CAD build for the part. Positions are in the model's coordinates, mm. Coordinates: 2 decimals unless noted, no trailing zeros. Order: outer loops, then holes, each group sorted by start corner. A loop starts at its lowest first (then second) coordinate and runs counter-clockwise, first axis right, second up. Notation, with made-up numbers: (11, 74.5) - (54, 74.5) arc R32 cw to (54, 113.5) - close; hole circle Ø10 at (59.5, 51). An arc over 180 degrees is marked (long way). Use one line per item in the form item = value.
```python
from build123d import *

# Parameters (mm, degrees)
F0_R     = 10
F1_DEPTH = 50
F2_DEPTH = 75
F3_SIZE  = 2


with BuildPart() as f1:
    # F0 (on Front) → F1 (new body)
    with BuildSketch(Plane.XZ):
        with BuildLine():
            ThreePointArc((2.083333, 24.913043), (18.399502, 16.92508), (25, 0))
            ThreePointArc((25, 0), (18.399502, -16.92508), (2.083333, -24.913043))
            Line((2.083333, -24.913043), (91.458333, -17.43913))
            ThreePointArc((91.458333, -17.43913), (72.5, 0), (91.458333, 17.43913))
            Line((91.458333, 17.43913), (2.083333, 24.913043))
        make_face()
        with BuildLine():
            ThreePointArc((2.083333, -24.913043), (18.399502, -16.92508), (25, 0))
            ThreePointArc((25, 0), (18.399502, 16.92508), (2.083333, 24.913043))
            ThreePointArc((2.083333, 24.913043), (-25, 0), (2.083333, -24.913043))
        make_face()
        Circle(F0_R, mode=Mode.SUBTRACT)
        with BuildLine():
            ThreePointArc((107.5, 0), (102.879651, 11.847556), (91.458333, 17.43913))
            ThreePointArc((91.458333, 17.43913), (72.5, 0), (91.458333, -17.43913))
            ThreePointArc((91.458333, -17.43913), (102.879651, -11.847556), (107.5, 0))
        make_face()
        with Locations((90, 0)):
            Circle(F0_R, mode=Mode.SUBTRACT)
    extrude(amount=F1_DEPTH)

    # F0 (on Front) → F2 (join)
    with BuildSketch(Plane.XZ):
        with BuildLine():
            ThreePointArc((2.083333, -24.913043), (18.399502, -16.92508), (25, 0))
            ThreePointArc((25, 0), (18.399502, 16.92508), (2.083333, 24.913043))
            ThreePointArc((2.083333, 24.913043), (-25, 0), (2.083333, -24.913043))
        make_face()
        Circle(F0_R, mode=Mode.SUBTRACT)
        with BuildLine():
            ThreePointArc((107.5, 0), (102.879651, 11.847556), (91.458333, 17.43913))
            ThreePointArc((91.458333, 17.43913), (72.5, 0), (91.458333, -17.43913))
            ThreePointArc((91.458333, -17.43913), (102.879651, -11.847556), (107.5, 0))
        make_face()
        with Locations((90, 0)):
            Circle(F0_R, mode=Mode.SUBTRACT)
    extrude(amount=F2_DEPTH)

    # F3
    f3_edges = [f1.edges().sort_by_distance(p)[0] for p in [
        (-10, -75, 0),
        (-2.083333, -75, 24.913043),
        (80, -75, 0),
        (88.541667, -75, 17.43913),
    ]]
    chamfer(f3_edges, length=F3_SIZE)


solid = f1.part
```
Item 1: Cut at B-B, the plane x = 0. Write the cut outline in (y, z).
Derived:
outline = (-75, -23) - (-73, -25) - (0, -25) - (0, -10) - (-73, -10) - (-75, -12) - close; (-75, 12) - (-73, 10) - (0, 10) - (0, 25) - (-73, 25) - (-75, 23) - close
Item 2: Drop flat-ended pins along their axis: pin 1 (1.5 mm diameter, centred on x = 27, y = -32.5, fed in from -Z); pin 2 (1.5 mm diameter, centred on y = -57.5, z = 11, fed in from +X); pin 3 (3 mm diameter, centred on x = 11, z = 1, fed in from +Y); pin 4 (5 mm diameter, centred on y = -66, z = 9, fed in from -X). Give the stop position or say it passes through.
Derived:
pin_1 = -22.89
pin_2 = 104.18
pin_3 = 0
pin_4 = -24.14
Item 3: Two-plate mould, pull along Z, no slides. Class faces 1 (the face through (80, -36, 0)), 2 (the face through (81.965, -73.125, -6.161)), 3 (the face through (47.396, -24.65, 21.124)), 4 (the face through (10, -75, -10)): +Z half, -Z half, draft (parallel to the pull), parting line (faces both ways), or undercut.
Derived:
face_1 = undercut
face_2 = undercut
face_3 = +Z half
face_4 = draft
Item 4: Drill centre lines: line 1 (Z direction, x = 90, y = -51); line 2 (Z direction, x = 0, y = -50); line 3 (X direction, y = -46, z = -1). Where is each one in solid material? Low to high. Write a range as [from, to].
Derived:
line_1 = [-17.5, -10], [10, 17.5]
line_2 = [-25, -10], [10, 25]
line_3 = [-24.98, -9.95], [9.95, 80.05], [99.95, 107.47]
Item 5: Cut at D-D, the plane x = 90. Write the cut outline in (y, z), plus the area to 3 significant figures.
Derived:
outline = (-75, -15.5) - (-73, -17.5) - (-50, -17.5) - (-50, -17.56) - (0, -17.56) - (0, -10) - (-73, -10) - (-75, -12) - close; (-75, 12) - (-73, 10) - (0, 10) - (0, 17.56) - (-50, 17.56) - (-50, 17.5) - (-73, 17.5) - (-75, 15.5) - close
area = 1,120 mm²
Item 6: Cut at C-C, the plane y = -41. Write the cut outline in (x, z), plus the area to 3 significant figures.
Derived:
outline = (2.08, -24.91) - (91.46, -17.44) arc R17.5 ccw to (91.46, 17.44) - (2.08, 24.91) arc R25 ccw (long way) to start; hole circle Ø20 at (0, 0); hole circle Ø20 at (90, 0)
area = 4,670 mm²
Item 7: Cut at A-A, the plane y = -54.5. Write the cut outline in (x, z), plus the area to 3 significant figures.
Derived:
outline = (2.08, -24.91) arc R25 ccw to (25, 0) arc R25 ccw to (2.08, 24.91) arc R25 ccw (long way) to start; circle Ø35 at (90, 0); hole circle Ø20 at (0, 0); hole circle Ø20 at (90, 0)
area = 2,300 mm²
